```python
from build123d import *

# Parameters (mm, degrees)
CROQUIS7_R              = 10.922
SALIENTE_EXTRUIR2_DEPTH = 13.614
CROQUIS8_R              = 1.2065
CORTAR_EXTRUIR3_DEPTH   = 13.614


with BuildPart() as part:
    # Croquis1 → Revolución1 (revolve)
    with BuildSketch(Plane.XY):
        with BuildLine():
            Line((-9.5, 0), (9.5, 0))
            ThreePointArc((9.5, 0), (0, 9.5), (-9.5, 0))
        make_face()
    revolve(axis=Axis((-9.5, 0, 0), (1, 0, 0)))

    # Croquis7 → Saliente-Extruir2 (add)
    with BuildSketch(Plane(origin=(0, 0, 0), x_dir=(1, 0, 0), z_dir=(0, 1, 0))):
        with Locations(Location((0, 0, 0), (0, 0, 270))):
            Circle(CROQUIS7_R)
    extrude(amount=SALIENTE_EXTRUIR2_DEPTH)

    # Croquis8 → Cortar-Extruir3 (cut)
    with BuildSketch(Plane(origin=(0, 13.614, 0), x_dir=(1, 0, 0), z_dir=(0, 1, 0))):
        with Locations(Location((-3.048, 0, 0), (0, 0, 270))):
            Circle(CROQUIS8_R)
        with Locations(Location((3.048, 0, 0), (0, 0, 90))):
            Circle(CROQUIS8_R)
    extrude(amount=-CORTAR_EXTRUIR3_DEPTH, mode=Mode.SUBTRACT)


solid = part.part
```
Work out the finished part from the listing and answer in its coordinate system (mm). A direction names the side the tool comes from. Give positions to 0.01 mm unless a question says otherwise; leave off trailing zeros. Order: outer loops, then holes, each group sorted by start corner. A loop starts at its lowest first (then second) coordinate and runs counter-clockwise, first axis right, second up.
1. For faces 1 (the flat face through (10, 0, 0)), 2 (the cylindrical face through (-4.118, 6.902, 0.557)), determine the directions among +Z, -Z, +X, -X, +Y, -Y from which every point of the face is accessible in a straight line to the end or side of a thin tool.
Result sheet:
face 1: -Y
face 2: +Y
2. Section D-D, the plane z = 5.75 is taken. Determine the outline of the cut face in (x, y).
Result sheet:
outline: (-9.29, 0) - (-7.56, 0) arc R7.56 ccw to (7.56, 0) - (9.29, 0) - (9.29, 13.61) - (-9.29, 13.61) - close
3. Section B-B, the plane x = 0 is taken. Determine the outline of the cut face in (y, z).
Result sheet:
outline: (0, -10.92) - (13.61, -10.92) - (13.61, 10.92) - (0, 10.92) - (0, 9.5) arc R9.5 ccw to (0, -9.5) - close
4. Straight lines are drawn through the part: L1, parallel to X at y = 4, z = 0; L2, parallel to X at y = 7, z = 0.5; L3, parallel to Y at x = 9.5, z = -4.5. For each, find the intervals that lie inside material, in ascending order.
Result sheet:
L1: x = -10.92 to -4.25, -1.84 to 1.84, 4.25 to 10.92
L2: x = -10.91 to -4.15, -1.95 to 1.95, 4.15 to 10.91
L3: y = 0 to 13.61
5. Each of these flat-tipped pins is pushed along its axis until it touches: P1, Ø1.5, axis at y = -6, z = -4.5, coming from the -X side; P2, Ø0.7, axis at x = 3, z = 0, coming from the +Y side; P3, Ø6, axis at x = -8, y = 4.5, coming from the -Z side. Where does it stop, or does it pass through?
Result sheet:
P1: stops at x = -6.68
P2: stops at y = 0
P3: stops at z = -9.71
6. The mould has two halves that part along X. Classify faces 3 (the flat face through (0, 13.614, 0)), 4 (the flat face through (-3, 0, 0)), 5 (the cylindrical face through (-4.18, 6.71, 10.09)), 6 (the flat face through (3, 0, 0)): released by +X, released by -X, zero draft, split by the parting line, or undercut.
Result sheet:
face 3: zero draft
face 4: undercut
face 5: split by the parting line
face 6: undercut
7. Section C-C, the plane y = -0.5 is taken. Determine the outline of the cut face in (x, z), and give its area (3 significant figures).
Result sheet:
outline: circle Ø18.97 at (0, 0)
area: 283 mm2
8. Section A-A, the plane z = 0 is taken. Determine the outline of the cut face in (x, y).
Result sheet:
outline: (-10.92, 0) - (-9.5, 0) arc R9.5 ccw to (9.5, 0) - (10.92, 0) - (10.92, 13.61) - (4.25, 13.61) - (4.25, 0) - (1.84, 0) - (1.84, 13.61) - (-1.84, 13.61) - (-1.84, 0) - (-4.25, 0) - (-4.25, 13.61) - (-10.92, 13.61) - close
